```python
from build123d import *

# Parameters (mm, degrees)
BASE_W               = 79
BASE_H               = 44
BASE_R               = 1.075
BOSS_EXTRUDE1_DEPTH  = 42
SHELL1_T             = -4.5
CUT_EXTRUDE2_START   = 4.5
BASE_7_R             = 1.075
CUT_EXTRUDE2_DEPTH   = 67.211020086
CUT_EXTRUDE3_START   = 2
BASE_8_R             = 1.075
CUT_EXTRUDE3_DEPTH   = 2
SKETCH3_W            = 26
SKETCH3_H            = 39.5
CUT_EXTRUDE4_DEPTH   = 23
FILLET1_R            = 2.5
CUT_EXTRUDE5_DEPTH   = 39.5
CUT_EXTRUDE6_DEPTH   = 74.5
FILLET2_R            = 1
MOUNT_R              = 1.625
CUT_EXTRUDE7_DEPTH   = 2.4
CUT_EXTRUDE8_START   = -2.25
CAMERA_MOUNT_HOLE_R  = 1
CUT_EXTRUDE8_DEPTH   = 75.777581073
FILLET2_OF_MIRROR3_R = 1


with BuildPart() as part:
    # Base → Boss-Extrude1 (new body)
    # profile 1 of 9: a face of its own
    with BuildSketch(Plane(origin=(0, 0, 0), x_dir=(1, 0, 0), z_dir=(0, 1, 0))):
        Rectangle(BASE_W, BASE_H)
        Polygon((27, -10.345299462), (27, -12.654700538), (29, -13.809401077), (31, -12.654700538), (31, -10.345299462), (29, -9.190598923), align=None, mode=Mode.SUBTRACT)
        Polygon((-31, -10.345299462), (-31, -12.654700538), (-29, -13.809401077), (-27, -12.654700538), (-27, -10.345299462), (-29, -9.190598923), align=None, mode=Mode.SUBTRACT)
        Polygon((-31, 12.654700538), (-31, 10.345299462), (-29, 9.190598923), (-27, 10.345299462), (-27, 12.654700538), (-29, 13.809401077), align=None, mode=Mode.SUBTRACT)
        Polygon((27, 12.654700538), (27, 10.345299462), (29, 9.190598923), (31, 10.345299462), (31, 12.654700538), (29, 13.809401077), align=None, mode=Mode.SUBTRACT)
    # profile 2 of 9: a face of its own
    with BuildSketch(Plane(origin=(0, 0, 0), x_dir=(1, 0, 0), z_dir=(0, 1, 0))):
        Polygon((-29, -9.190598923), (-31, -10.345299462), (-31, -12.654700538), (-29, -13.809401077), (-27, -12.654700538), (-27, -10.345299462), align=None)
        with Locations((-29, -11.5)):
            Circle(BASE_R, mode=Mode.SUBTRACT)
    # profile 3 of 9: a face of its own
    with BuildSketch(Plane(origin=(0, 0, 0), x_dir=(1, 0, 0), z_dir=(0, 1, 0))):
        with Locations((-29, -11.5)):
            Circle(BASE_R)
    # profile 4 of 9: a face of its own
    with BuildSketch(Plane(origin=(0, 0, 0), x_dir=(1, 0, 0), z_dir=(0, 1, 0))):
        Polygon((-29, 13.809401077), (-31, 12.654700538), (-31, 10.345299462), (-29, 9.190598923), (-27, 10.345299462), (-27, 12.654700538), align=None)
        with Locations((-29, 11.5)):
            Circle(BASE_R, mode=Mode.SUBTRACT)
    # profile 5 of 9: a face of its own
    with BuildSketch(Plane(origin=(0, 0, 0), x_dir=(1, 0, 0), z_dir=(0, 1, 0))):
        with Locations((-29, 11.5)):
            Circle(BASE_R)
    # profile 6 of 9: a face of its own
    with BuildSketch(Plane(origin=(0, 0, 0), x_dir=(1, 0, 0), z_dir=(0, 1, 0))):
        Polygon((29, -9.190598923), (27, -10.345299462), (27, -12.654700538), (29, -13.809401077), (31, -12.654700538), (31, -10.345299462), align=None)
        with Locations((29, -11.5)):
            Circle(BASE_R, mode=Mode.SUBTRACT)
    # profile 7 of 9: a face of its own
    with BuildSketch(Plane(origin=(0, 0, 0), x_dir=(1, 0, 0), z_dir=(0, 1, 0))):
        with Locations((29, -11.5)):
            Circle(BASE_R)
    # profile 8 of 9: a face of its own
    with BuildSketch(Plane(origin=(0, 0, 0), x_dir=(1, 0, 0), z_dir=(0, 1, 0))):
        Polygon((29, 13.809401077), (27, 12.654700538), (27, 10.345299462), (29, 9.190598923), (31, 10.345299462), (31, 12.654700538), align=None)
        with Locations((29, 11.5)):
            Circle(BASE_R, mode=Mode.SUBTRACT)
    # profile 9 of 9: a face of its own
    with BuildSketch(Plane(origin=(0, 0, 0), x_dir=(1, 0, 0), z_dir=(0, 1, 0))):
        with Locations((29, 11.5)):
            Circle(BASE_R)
    extrude(amount=BOSS_EXTRUDE1_DEPTH)

    # Shell1
    shell1_openings = [part.faces().sort_by_distance(p)[0] for p in [
        (0, 42, 0),
    ]]
    offset(amount=SHELL1_T, openings=shell1_openings, kind=Kind.INTERSECTION)

    # Base<7> → Cut-Extrude2 (cut, through all)
    with BuildSketch(Plane(origin=(0, 0, 0), x_dir=(1, 0, 0), z_dir=(0, 1, 0)).offset(CUT_EXTRUDE2_START)):
        with Locations(Location((-29, -11.5, 0), (0, 0, 270))):
            Circle(BASE_7_R)
        with Locations(Location((-29, 11.5, 0), (0, 0, 270))):
            Circle(BASE_7_R)
        with Locations(Location((29, -11.5, 0), (0, 0, 270))):
            Circle(BASE_7_R)
        with Locations(Location((29, 11.5, 0), (0, 0, 270))):
            Circle(BASE_7_R)
    extrude(amount=-CUT_EXTRUDE2_DEPTH, mode=Mode.SUBTRACT)

    # Base<8> → Cut-Extrude3 (cut)
    # profile 1 of 4: a face of its own
    with BuildSketch(Plane(origin=(0, 0, 0), x_dir=(1, 0, 0), z_dir=(0, 1, 0)).offset(CUT_EXTRUDE3_START)):
        Polygon((29, 13.809401077), (27, 12.654700538), (27, 10.345299462), (29, 9.190598923), (31, 10.345299462), (31, 12.654700538), align=None)
        with Locations(Location((29, 11.5, 0), (0, 0, 270))):
            Circle(BASE_8_R, mode=Mode.SUBTRACT)
    # profile 2 of 4: a face of its own
    with BuildSketch(Plane(origin=(0, 0, 0), x_dir=(1, 0, 0), z_dir=(0, 1, 0)).offset(CUT_EXTRUDE3_START)):
        Polygon((29, -9.190598923), (27, -10.345299462), (27, -12.654700538), (29, -13.809401077), (31, -12.654700538), (31, -10.345299462), align=None)
        with Locations(Location((29, -11.5, 0), (0, 0, 270))):
            Circle(BASE_8_R, mode=Mode.SUBTRACT)
    # profile 3 of 4: a face of its own
    with BuildSketch(Plane(origin=(0, 0, 0), x_dir=(1, 0, 0), z_dir=(0, 1, 0)).offset(CUT_EXTRUDE3_START)):
        Polygon((-29, -9.190598923), (-31, -10.345299462), (-31, -12.654700538), (-29, -13.809401077), (-27, -12.654700538), (-27, -10.345299462), align=None)
        with Locations(Location((-29, -11.5, 0), (0, 0, 270))):
            Circle(BASE_8_R, mode=Mode.SUBTRACT)
    # profile 4 of 4: a face of its own
    with BuildSketch(Plane(origin=(0, 0, 0), x_dir=(1, 0, 0), z_dir=(0, 1, 0)).offset(CUT_EXTRUDE3_START)):
        Polygon((-29, 13.809401077), (-31, 12.654700538), (-31, 10.345299462), (-29, 9.190598923), (-27, 10.345299462), (-27, 12.654700538), align=None)
        with Locations(Location((-29, 11.5, 0), (0, 0, 270))):
            Circle(BASE_8_R, mode=Mode.SUBTRACT)
    extrude(amount=-CUT_EXTRUDE3_DEPTH, mode=Mode.SUBTRACT)

    # Sketch3 → Cut-Extrude4 (cut)
    with BuildSketch(Plane(origin=(0, 42, 0), x_dir=(1, 0, 0), z_dir=(0, 1, 0))):
        Rectangle(SKETCH3_W, SKETCH3_H)
    extrude(amount=-CUT_EXTRUDE4_DEPTH, mode=Mode.SUBTRACT)

    # Fillet1
    fillet1_edges = [part.edges().sort_by_distance(p)[0] for p in [
        (39.5, 21, 22),
        (-39.5, 21, 22),
        (-39.5, 21, -22),
        (39.5, 21, -22),
    ]]
    fillet(fillet1_edges, radius=FILLET1_R)

    # INPUTS → Cut-Extrude5 (cut)
    with BuildSketch(Plane.XY.offset(22)):
        Polygon((-35, 17), (-34, 4.5), (34, 4.5), (35, 17), align=None)
    cut_extrude5 = extrude(amount=-CUT_EXTRUDE5_DEPTH, mode=Mode.SUBTRACT)

    # SD_CARD → Cut-Extrude6 (cut)
    with BuildSketch(Plane.ZY.offset(39.5)):
        with BuildLine():
            Line((-16, 4.5), (16, 4.5))
            ThreePointArc((16, 4.5), (17.060660172, 4.939339828), (17.5, 6))
            Line((17.5, 6), (17.5, 23))
            ThreePointArc((17.5, 23), (17.060660172, 24.060660172), (16, 24.5))
            Line((16, 24.5), (-16, 24.5))
            ThreePointArc((-16, 24.5), (-17.060660172, 24.060660172), (-17.5, 23))
            Line((-17.5, 23), (-17.5, 6))
            ThreePointArc((-17.5, 6), (-17.060660172, 4.939339828), (-16, 4.5))
        make_face()
    cut_extrude6 = extrude(amount=-CUT_EXTRUDE6_DEPTH, mode=Mode.SUBTRACT)

    # Fillet2
    fillet2_edges = [part.edges().sort_by_distance(p)[0] for p in [
        (34, 4.5, 19.75),
        (35, 17, 19.75),
        (-35, 17, 19.75),
        (-34, 4.5, 19.75),
    ]]
    fillet(fillet2_edges, radius=FILLET2_R)

    # Mirror1: Cut-Extrude6 across plane
    add(cut_extrude6.mirror(Plane.ZY), mode=Mode.SUBTRACT)

    # Mount → Cut-Extrude7 (cut)
    with BuildSketch(Plane(origin=(0, 42, 0), x_dir=(1, 0, 0), z_dir=(0, 1, 0))):
        with Locations(Location((-37, 19.5, 0), (0, 0, 270))):
            Circle(MOUNT_R)
        with Locations(Location((37, 19.5, 0), (0, 0, 270))):
            Circle(MOUNT_R)
        with Locations(Location((37, -19.5, 0), (0, 0, 270))):
            Circle(MOUNT_R)
        with Locations(Location((-37, -19.5, 0), (0, 0, 270))):
            Circle(MOUNT_R)
    extrude(amount=-CUT_EXTRUDE7_DEPTH, mode=Mode.SUBTRACT)

    # Camera_Mount_Hole → Cut-Extrude8 (cut)
    with BuildSketch(Plane.XY.offset(22).offset(CUT_EXTRUDE8_START)):
        with Locations((0, 21.5)):
            Circle(CAMERA_MOUNT_HOLE_R)
    cut_extrude8 = extrude(amount=CUT_EXTRUDE8_DEPTH, mode=Mode.SUBTRACT)

    # Mirror2: Cut-Extrude8 across plane
    add(cut_extrude8.mirror(Plane.XY), mode=Mode.SUBTRACT)

    # Mirror3: Cut-Extrude5 across plane
    add(cut_extrude5.mirror(Plane.XY), mode=Mode.SUBTRACT)

    # Fillet2 of Mirror3
    fillet2_of_mirror3_edges = [part.edges().sort_by_distance(p)[0] for p in [
        (34, 4.5, -19.75),
        (35, 17, -19.75),
        (-35, 17, -19.75),
        (-34, 4.5, -19.75),
    ]]
    fillet(fillet2_of_mirror3_edges, radius=FILLET2_OF_MIRROR3_R)


solid = part.part
```
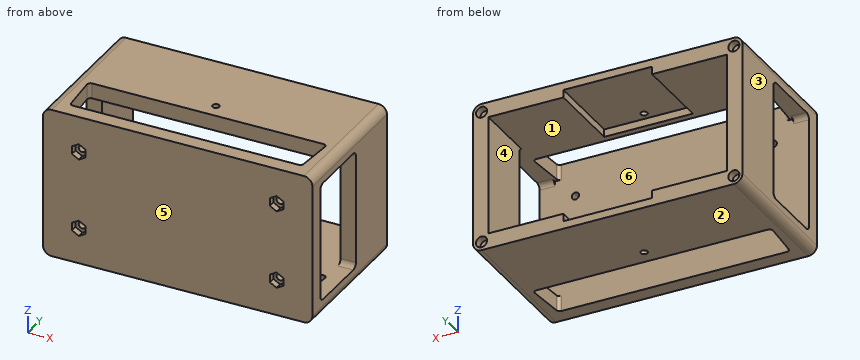
Work out the finished part from the listing and answer in its coordinate system (mm). Face numbers are marked on the shaded views. A direction names the side the tool comes from. Give positions to 0.01 mm unless a question says otherwise; leave off trailing zeros. Write each loop counter-clockwise with the first axis right and the second up, starting at its lowest first coordinate (ties: lowest second). Pieces come first, ordered by that corner, then holes.
(1) Which of the six approach directions +Z, -Z, +X, -X, +Y, -Y give full straight-line access (tool end or side, diameter ignored) to the marked faces 4, 5 and 6?
Final values:
face 4: +Y
face 5: +Z, -Z, +X, -X, -Y
face 6: none
(2) The part is cut by section B-B on y = 12.5. Write down the section's boundary in (x, z).
Final values:
outline: (-39.5, -19.5) arc R2.5 ccw to (-37, -22) - (-34.64, -22) - (-34.64, -17.5) - (-39.5, -17.5) - close; (-39.5, 17.5) - (-34.64, 17.5) - (-34.64, 22) - (-37, 22) arc R2.5 ccw to (-39.5, 19.5) - close; (34.64, -22) - (37, -22) arc R2.5 ccw to (39.5, -19.5) - (39.5, -17.5) - (34.64, -17.5) - close; (34.64, 17.5) - (39.5, 17.5) - (39.5, 19.5) arc R2.5 ccw to (37, 22) - (34.64, 22) - close
(3) The part is cut by section A-A on x = 19.5. Write down the section's boundary in (y, z).
Final values:
outline: (0, -22) - (4.5, -22) - (4.5, 22) - (0, 22) - close; (17, -22) - (42, -22) - (42, -17.5) - (17, -17.5) - close; (17, 17.5) - (42, 17.5) - (42, 22) - (17, 22) - close
(4) Straight lines are drawn through the part: line 1 (Y direction, x = 0, z = 21.5); line 2 (Z direction, x = 32, y = 31); line 3 (X direction, y = 40.4, z = 19.5) (3 decimals). For each, find the intervals that lie inside material, in ascending order.
Final values:
line 1: y = 0 to 4.5, 17 to 20.5, 22.5 to 42
line 2: z = -22 to -17.5, 17.5 to 22
line 3: x = -39.5 to -38.625, -35.375 to -13, 13 to 35.375, 38.625 to 39.5
(5) The part is cut by section C-C on x = 0. Write down the section's boundary in (y, z), plus the area to 4 significant figures.
Final values:
outline: (0, -22) - (4.5, -22) - (4.5, 22) - (0, 22) - close; (17, -22) - (20.5, -22) - (20.5, -19.75) - (19, -19.75) - (19, -17.5) - (17, -17.5) - close; (17, 17.5) - (19, 17.5) - (19, 19.75) - (20.5, 19.75) - (20.5, 22) - (17, 22) - close; (22.5, -22) - (42, -22) - (42, -19.75) - (22.5, -19.75) - close; (22.5, 19.75) - (42, 19.75) - (42, 22) - (22.5, 22) - close
area: 310.5 mm2
(6) The part is cut by section D-D on z = -0.5. Write down the section's boundary in (x, y).
Final values:
outline: (-39.5, 0) - (39.5, 0) - (39.5, 4.5) - (-39.5, 4.5) - close; (-39.5, 24.5) - (-35, 24.5) - (-35, 42) - (-39.5, 42) - close; (35, 24.5) - (39.5, 24.5) - (39.5, 42) - (35, 42) - close
(7) Flat-ended cylindrical pins translate along their axes: pin 1 Ø3 at (x, z) = (37, -19.5) entering from +Y; pin 2 Ø2 at (x, y) = (12, 15.5) entering from -Z. Find the tip coordinate at first contact, or state that the pin passes through.
Final values:
pin 1: stops at y = 39.6
pin 2: passes through
(8) The mould has two halves that part along Z. Classify the marked faces 1, 2 and 3: pulls with the +Z half, pulls with the -Z half, needs draft (parallel to the pull), parting line crosses it, or undercut.
Final values:
face 1: undercut
face 2: pulls with the -Z half
face 3: needs draft
